Geometry: final body of the model. Coordinates: model frame, mm. Round coordinates to 2 decimals unless told otherwise and drop trailing zeros. Loops run counter-clockwise (first coordinate to the right, second up) from the corner with the lowest first, then second, coordinate; pieces in that order, holes last. Notation, with made-up numbers: M 72,62 L 90,62 A27 cw 90,92 Z; hole C -10.5,89.5 d10. An arc over 180 degrees is marked long. Answer as a JSON object with one key per item and string values.
Autodesk Inventor part; units mm, degrees
ref_plane "Start Plane" through (0, 0, 0) normal (0, 0, 1) x (1, 0, 0)
ref_plane "End Plane" through (0, 0, 10) normal (0, 0, 1) x (1, 0, 0)
ref_plane "YZ Plane" through (0, 0, 0) normal (1, 0, 0) x (0, 1, 0)
ref_plane "Start Plane" through (0, 0, 0) normal (0, 0, 1) x (1, 0, 0)
ref_plane "End Plane" through (0, 0, 10) normal (0, 0, 1) x (1, 0, 0)
sketch "Sketch3" plane through (0, 0, 0) normal (0, 0, 1) x (1, 0, 0)
  line L0 (0, 0) -> (0, 10) construction
  line L1 (-10, 10) -> (-10, 0) construction
  line L2 (0, 0) -> (-10, 0) construction
  circle A0 centre (-10, 0) radius 2.1
  line L3 (-13.9007, 3.9007) -> (-6.0993, 3.9007) construction
  line L4 (-6.0993, 3.9007) -> (-6.0993, -3.9007) construction
  line L5 (-6.0993, -3.9007) -> (-13.9007, -3.9007) construction
  line L6 (-13.9007, -3.9007) -> (-13.9007, 3.9007) construction
  line L7 (-13.9007, 3.9007) -> (-6.0993, -3.9007) construction
  line L8 (-6.0993, 3.9007) -> (-13.9007, -3.9007) construction
  line L9 (-13.9007, -2.84) -> (-12.84, -3.9007) construction
  line L10 (-13.9007, -2.84) -> (-12.4007, -2.84) construction
  line L11 (-12.84, -3.9007) -> (-15.4993, -6.56)
  line L12 (-15.4993, -6.56) -> (-15.4993, -8.2)
  line L13 (-15.4993, -8.2) -> (-12.84, -8.2)
  line L14 (-12.84, -8.2) -> (-14.64, -10)
  line L15 (-7.16, -3.9007) -> (-4.5007, -6.56)
  line L16 (-4.5007, -6.56) -> (-4.5007, -8.2)
  line L17 (-4.5007, -8.2) -> (-7.16, -8.2)
  line L18 (-7.16, -8.2) -> (-5.36, -10)
  line L19 (-12.84, -3.9007) -> (-7.16, -3.9007)
  line L20 (-12.84, 3.9007) -> (-13.9007, 2.84) construction
  line L21 (-12.84, 3.9007) -> (-12.84, 2.4007) construction
  line L22 (-13.9007, 2.84) -> (-16.56, 5.4993)
  line L23 (-16.56, 5.4993) -> (-18.2, 5.4993)
  line L24 (-18.2, 5.4993) -> (-18.2, 2.84)
  line L25 (-18.2, 2.84) -> (-20, 4.64)
  line L26 (-18.2, -2.84) -> (-20, -4.64)
  line L27 (-18.2, -5.4993) -> (-18.2, -2.84)
  line L28 (-16.56, -5.4993) -> (-18.2, -5.4993)
  line L29 (-13.9007, -2.84) -> (-16.56, -5.4993)
  line L30 (-13.9007, 2.84) -> (-13.9007, -2.84)
  line L31 (-6.0993, 2.84) -> (-7.16, 3.9007) construction
  line L32 (-6.0993, 2.84) -> (-7.5993, 2.84) construction
  line L33 (-7.16, 3.9007) -> (-4.5007, 6.56)
  line L34 (-4.5007, 6.56) -> (-4.5007, 8.2)
  line L35 (-4.5007, 8.2) -> (-7.16, 8.2)
  line L36 (-7.16, 8.2) -> (-5.36, 10)
  line L37 (-12.84, 8.2) -> (-14.64, 10)
  line L38 (-15.4993, 8.2) -> (-12.84, 8.2)
  line L39 (-15.4993, 6.56) -> (-15.4993, 8.2)
  line L40 (-12.84, 3.9007) -> (-15.4993, 6.56)
  line L41 (-7.16, 3.9007) -> (-12.84, 3.9007)
  line L42 (-6.0993, 2.84) -> (-2.6993, 6.24)
  line L43 (-2.6993, 6.24) -> (-2.6993, 8.2)
  line L44 (-4.5007, 8.2) -> (0, 8.2) construction
  line L45 (-6.0993, -2.84) -> (-2.6993, -6.24)
  line L46 (-2.6993, -6.24) -> (-2.6993, -8.2)
  line L47 (10, 10) -> (10, 0) construction
  circle A1 centre (10, 0) radius 2.1
  line L48 (13.9007, 3.9007) -> (6.0993, -3.9007) construction
  line L49 (13.9007, -2.84) -> (12.84, -3.9007) construction
  line L50 (12.84, -3.9007) -> (15.4993, -6.56)
  line L51 (15.4993, -6.56) -> (15.4993, -8.2)
  line L52 (15.4993, -8.2) -> (12.84, -8.2)
  line L53 (12.84, -8.2) -> (14.64, -10)
  line L54 (7.16, -8.2) -> (5.36, -10)
  line L55 (4.5007, -8.2) -> (7.16, -8.2)
  line L56 (4.5007, -6.56) -> (4.5007, -8.2)
  line L57 (7.16, -3.9007) -> (4.5007, -6.56)
  line L58 (12.84, -3.9007) -> (7.16, -3.9007)
  line L59 (13.9007, 2.84) -> (13.9007, -2.84)
  line L60 (13.9007, 2.84) -> (16.56, 5.4993)
  line L61 (16.56, 5.4993) -> (18.2, 5.4993)
  line L62 (18.2, 5.4993) -> (18.2, 2.84)
  line L63 (18.2, 2.84) -> (20, 4.64)
  line L64 (18.2, -5.4993) -> (18.2, -2.84)
  line L65 (18.2, -2.84) -> (20, -4.64)
  line L66 (16.56, -5.4993) -> (18.2, -5.4993)
  line L67 (13.9007, -2.84) -> (16.56, -5.4993)
  line L68 (7.16, 3.9007) -> (12.84, 3.9007)
  line L69 (7.16, 3.9007) -> (4.5007, 6.56)
  line L70 (4.5007, 6.56) -> (4.5007, 8.2)
  line L71 (4.5007, 8.2) -> (7.16, 8.2)
  line L72 (7.16, 8.2) -> (5.36, 10)
  line L73 (15.4993, 8.2) -> (12.84, 8.2)
  line L74 (12.84, 8.2) -> (14.64, 10)
  line L75 (15.4993, 6.56) -> (15.4993, 8.2)
  line L76 (12.84, 3.9007) -> (15.4993, 6.56)
  line L77 (6.0993, 2.84) -> (2.6993, 6.24)
  line L78 (2.6993, 6.24) -> (2.6993, 8.2)
  line L79 (6.0993, -2.84) -> (2.6993, -6.24)
  line L80 (2.6993, -6.24) -> (2.6993, -8.2)
  line L81 (-14.64, -10) -> (-18.2, -10)
  line L82 (-20, -8.2) -> (-20, -4.64)
  line L83 (-20, 4.64) -> (-20, 8.2)
  line L84 (-18.2, 10) -> (-14.64, 10)
  line L85 (18.2, -10) -> (14.64, -10)
  line L86 (5.36, -10) -> (-5.36, -10)
  line L87 (-5.36, 10) -> (5.36, 10)
  line L88 (14.64, 10) -> (18.2, 10)
  line L89 (20, 8.2) -> (20, 4.64)
  line L90 (20, -4.64) -> (20, -8.2)
  line L91 (-2.6993, -8.2) -> (2.6993, -8.2)
  line L92 (-2.6993, 8.2) -> (2.6993, 8.2)
  line L93 (-6.0993, 2.84) -> (-6.0993, -2.84)
  line L94 (6.0993, 2.84) -> (6.0993, -2.84)
  arc A2 (-20, -8.2) -> (-18.2, -10) centre (-18.2, -8.2) ccw
  arc A3 (-18.2, 10) -> (-20, 8.2) centre (-18.2, 8.2) ccw
  arc A4 (18.2, -10) -> (20, -8.2) centre (18.2, -8.2) ccw
  arc A5 (20, 8.2) -> (18.2, 10) centre (18.2, 8.2) ccw
  point P0 (-13.9007, -3.9007)
  point P1 (-13.9007, 3.9007)
  point P2 (-13.9007, 3.9007)
  point P3 (-6.0993, 3.9007)
  point P4 (6.0993, 3.9007)
  point P5 (13.9007, -3.9007)
  point P6 (12.4007, -2.84)
  point P7 (13.9007, -3.9007)
  point P8 (13.9007, 3.9007)
  point P9 (12.84, 3.9007)
  point P10 (12.84, 2.4007)
  point P11 (13.9007, 3.9007)
  point P12 (6.0993, 3.9007)
  point P13 (7.5993, 2.84)
  point P14 (-20, 10)
  point P15 (20, -10)
  point P16 (20, 10)
  point P17 (-20, -10)
  dimension "d26" = 10
  dimension "d27" = 10
  dimension "d28" = 4.2
  dimension "d29" = 1.5
  dimension "d30" = 45
  dimension "d32" = 45
  dimension "d33" = 1.64
  dimension "d34" = 1.8
  dimension "d35" = 10
  dimension "d36" = 5.68
  dimension "d39" = 180
  dimension "d41" = 1.96
  dimension "d42" = 5.68
  dimension "d45" = 1.8
extrude "Body" add sketch "Sketch3" along normal blind 250
sketch "Sketch4" plane through (0, 0, 0) normal (0, 0, 1) x (1, 0, 0)
  line L0 (0, 0) -> (10, 0)
ref_plane "Work Plane3" through (0, 0, 0) normal (0, -1, 0) x (1, 0, 0)
sketch "Sketch5" plane through (0, 0, 0) normal (0, -1, 0) x (1, 0, 0)
  line L0 (-2, 0) -> (12, 0)
  line L1 (-2, 10) -> (12, 10)
  dimension "d51" = 10
equation "\"d42\" = d36"
equation "\"G_OFFSET_START\" = 0"
equation "\"G_OFFSET_END\" = 0"
equation "\"G_L\" = d51"
properties part number "vslot 20 x 40" material "Aluminum 6061"
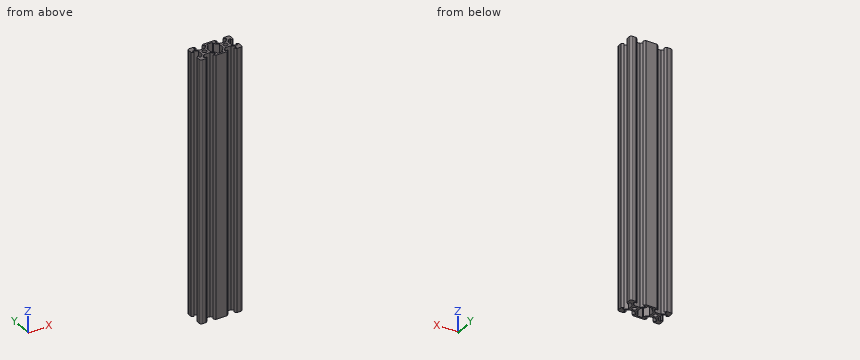
1) Cut plane A-A on y = 0. Return the cut outline in (x, z), and give its area (3 significant figures).
Geometry results:
{"outline": "M -13.9,0 L -12.1,0 L -12.1,250 L -13.9,250 Z; M -7.9,0 L -6.1,0 L -6.1,250 L -7.9,250 Z; M 6.1,0 L 7.9,0 L 7.9,250 L 6.1,250 Z; M 12.1,0 L 13.9,0 L 13.9,250 L 12.1,250 Z", "area": "1,800 mm2"}
2) Line query: probe 1 along Y at (x, z) = (0.5, 162.5); probe 2 along Y at (x, z) = (14, 144.5); probe 3 along X at (y, z) = (4.75, 160). Output: solid intervals per line, ascending.
Geometry results:
{"probe 1": "-10 to -8.2, 8.2 to 10", "probe 2": "-9.36 to -8.2, -5.06 to -2.94, 2.94 to 5.06, 8.2 to 9.36", "probe 3": "-20 to -18.2, -15.81 to -13.69, -6.31 to -4.19, 4.19 to 6.31, 13.69 to 15.81, 18.2 to 20"}
3) Cut plane C-C on x = -10. Return the cut outline in (y, z), and give its area (3 significant figures).
Geometry results:
{"outline": "M -3.9,0 L -2.1,0 L -2.1,250 L -3.9,250 Z; M 2.1,0 L 3.9,0 L 3.9,250 L 2.1,250 Z", "area": "900 mm2"}
4) First-contact query: pin 1 (8 mm diameter, centred on x = -14, z = 174.5, fed in from +Y); pin 2 (2 mm diameter, centred on x = -11.5, y = -5, fed in from -Z); pin 3 (1 mm diameter, centred on x = -13.5, z = 63.5, fed in from -Y); pin 4 (4 mm diameter, centred on y = 2, z = 33, fed in from +X). Flat tips, straight axial feed; report the tip coordinate or a pass-through.
Geometry results:
{"pin 1": "y = 10", "pin 2": "through", "pin 3": "y = -9.36", "pin 4": "x = 19.36"}
5) Cut plane D-D on z = 122.5. Count the separate pieces of the cut face and the enclosed holes in it, and give its area (3 significant figures).
Geometry results:
{"separate pieces": "1", "enclosed holes": "3", "area": "297 mm2"}
6) Cut plane B-B on x = 0.5. Return the cut outline in (y, z).
Geometry results:
{"outline": "M -10,0 L -8.2,0 L -8.2,250 L -10,250 Z; M 8.2,0 L 10,0 L 10,250 L 8.2,250 Z"}
